from build123d import *

# Parameters (mm, degrees)
SKETCH1_W           = 35.5
SKETCH1_H           = 32
BOSS_EXTRUDE1_DEPTH = 1.66
SKETCH2_W           = 31.32
SKETCH2_H           = 15.62
BOSS_EXTRUDE2_DEPTH = 1


with BuildPart() as part:
    # Sketch1 → Boss-Extrude1 (new body)
    with BuildSketch(Plane.XY):
        with Locations((17.75, 16)):
            Rectangle(SKETCH1_W, SKETCH1_H)
        with BuildLine():
            Line((4.5, 30.95), (5.6, 30.95))
            ThreePointArc((5.6, 30.95), (6.7, 29.85), (5.6, 28.75))
            Line((5.6, 28.75), (4.5, 28.75))
            ThreePointArc((4.5, 28.75), (3.4, 29.85), (4.5, 30.95))
        make_face(mode=Mode.SUBTRACT)
        with BuildLine():
            Line((29.9, 28.75), (31, 28.75))
            ThreePointArc((31, 28.75), (32.1, 29.85), (31, 30.95))
            Line((31, 30.95), (29.9, 30.95))
            ThreePointArc((29.9, 30.95), (28.8, 29.85), (29.9, 28.75))
        make_face(mode=Mode.SUBTRACT)
        with BuildLine():
            Line((29.9, 1.05), (31, 1.05))
            ThreePointArc((31, 1.05), (32.1, 2.15), (31, 3.25))
            Line((31, 3.25), (29.9, 3.25))
            ThreePointArc((29.9, 3.25), (28.8, 2.15), (29.9, 1.05))
        make_face(mode=Mode.SUBTRACT)
        with BuildLine():
            Line((4.5, 1.05), (5.6, 1.05))
            ThreePointArc((5.6, 1.05), (6.7, 2.15), (5.6, 3.25))
            Line((5.6, 3.25), (4.5, 3.25))
            ThreePointArc((4.5, 3.25), (3.4, 2.15), (4.5, 1.05))
        make_face(mode=Mode.SUBTRACT)
    extrude(amount=BOSS_EXTRUDE1_DEPTH)

    # Sketch2 → Boss-Extrude2 (add)
    with BuildSketch(Plane.XY):
        with Locations((17.75, 18.05)):
            Rectangle(SKETCH2_W, SKETCH2_H)
    extrude(amount=-BOSS_EXTRUDE2_DEPTH)


solid = part.part
Verification items for the finished model (mm, model axes). A direction names the side the tool comes from. Coordinates: 2 decimals unless noted, no trailing zeros. Write each loop counter-clockwise with the first axis right and the second up, starting at its lowest first coordinate (ties: lowest second). Pieces come first, ordered by that corner, then holes. Notation, with made-up numbers: (16.25, -5.75) -> (72.25, -5.75) arc R5 cw to (72.25, 2.25) -> close; hole circle Ø10 at (88.5, -9.5). An arc over 180 degrees is marked (long way). One line per item, written item: value. Start each with the question number.
Q1. Cross-section at C-C on y = 19. Enter the section's corners in (x, z).
Q2. Cross-section at A-A on y = 2.15. Enter the section's corners in (x, z), and give its area (3 significant figures).
Q3. Go/stop test with flat-tipped pins: P1, Ø0.8, axis at x = 14, z = -0.5, coming from the -Y side; P2, Ø0.5, axis at y = 20, z = -0.5, coming from the +X side; P3, Ø0.5, axis at y = 20, z = -0.5, coming from the -X side. Record where each tip stops, or that it passes through.
Q4. Mould release check, pull along X, two halves, no side actions. Record for faces 1 (the flat face through (0, 16, 1)), 2 (the cylindrical face through (28.8, 2.2, 0.8)), 3 (the flat face through (17.5, 10.24, -0.5)), 4 (the flat face through (33.41, 17.9, -0.5)): pulls with the +X half, pulls with the -X half, needs draft (parallel to the pull), parting line crosses it, or undercut.
Q5. Cross-section at B-B on z = 0.55. Enter the section's corners in (x, y).
Q6. Cross-section at D-D on x = 3. Enter the section's corners in (y, z).
Q7. Thickness scan on L1, parallel to Y at x = 30, z = 0.6; L2, parallel to X at y = 2, z = 1.2; L3, parallel to Z at x = 18.5, y = 3.5. Record the ranges inside material, lowest first. Write a range as from..to.
Q8. Access from +Z, -Z, +X, -X, +Y, -Y to the whole of each face (thin tool, end or side, straight path). Record for faces 5 (the flat face through (18, 18, -1)), 6 (the flat face through (2.09, 17.9, -0.5)), 7 (the flat face through (17.5, 25.86, -0.5)), 8 (the cylindrical face through (3.4, 29.8, 0.8)).
Checked values:
1. outline: (0, 0) -> (2.09, 0) -> (2.09, -1) -> (33.41, -1) -> (33.41, 0) -> (35.5, 0) -> (35.5, 1.66) -> (0, 1.66) -> close
2. outline: (0, 0) -> (3.4, 0) -> (3.4, 1.66) -> (0, 1.66) -> close; (6.7, 0) -> (28.8, 0) -> (28.8, 1.66) -> (6.7, 1.66) -> close; (32.1, 0) -> (35.5, 0) -> (35.5, 1.66) -> (32.1, 1.66) -> close
2. area: 48.0 mm²
3. P1: stops at y = 10.24
3. P2: stops at x = 33.41
3. P3: stops at x = 2.09
4. face 1: pulls with the -X half
4. face 2: undercut
4. face 3: needs draft
4. face 4: pulls with the +X half
5. outline: (0, 0) -> (35.5, 0) -> (35.5, 32) -> (0, 32) -> close; hole (4.5, 1.05) -> (5.6, 1.05) arc R1.1 ccw to (5.6, 3.25) -> (4.5, 3.25) arc R1.1 ccw to start; hole (4.5, 28.75) -> (5.6, 28.75) arc R1.1 ccw to (5.6, 30.95) -> (4.5, 30.95) arc R1.1 ccw to start; hole (29.9, 1.05) -> (31, 1.05) arc R1.1 ccw to (31, 3.25) -> (29.9, 3.25) arc R1.1 ccw to start; hole (29.9, 28.75) -> (31, 28.75) arc R1.1 ccw to (31, 30.95) -> (29.9, 30.95) arc R1.1 ccw to start
6. outline: (0, 0) -> (10.24, 0) -> (10.24, -1) -> (25.86, -1) -> (25.86, 0) -> (32, 0) -> (32, 1.66) -> (0, 1.66) -> close
7. L1: y = 0..1.05, 3.25..28.75, 30.95..32
7. L2: x = 0..3.41, 6.69..28.81, 32.09..35.5
7. L3: z = 0..1.66
8. face 5: -Z, +X, -X, +Y, -Y
8. face 6: -Z, -X, +Y, -Y
8. face 7: -Z, +X, -X, +Y
8. face 8: +Z, -Z
